The model under review builds one solid part; all positions refer to its coordinate system, in mm. A direction names the side the tool comes from. Round coordinates to 2 decimals unless told otherwise and drop trailing zeros. Write each loop counter-clockwise with the first axis right and the second up, starting at its lowest first coordinate (ties: lowest second). Pieces come first, ordered by that corner, then holes. Notation, with made-up numbers: M -22,21 L 26,21 A30 ccw 26,44 Z; hole C 7,12.25 d3. An arc over 180 degrees is marked long. One line per item, written item: value. Start each with the question number.
1) Take a section at B-B, the plane x = 3. Write out the cut boundary in (y, z), and give its area (3 significant figures).
2) Take a section at D-D, the plane z = 11. Write out the cut boundary in (x, y).
3) Tool access review of faces 1 (the face through (0, 60, -1)), 2 (the face through (1.054, 15.789, -13.672)), 3 (the face through (-4.6, 45.07, 17.19)), 4 (the face through (0, 43, -15)), 5 (the face through (2, 30, 16)): name each direction out of +Z, -Z, +X, -X, +Y, -Y from which nothing blocks a thin tool from reaching the whole face with its end or side.
4) Mouldability with a two-part tool opening along X and no side actions: class faces 6 (the face through (0, 15, -21)), 7 (the face through (10, 31, -1)), 8 (the face through (0.05, 23.03, -6.25)) as +X half, -X half, draft (parallel to the pull), parting line (faces both ways), or undercut.
5) Wall thickness on probe 1 along X at (y, z) = (59, -5); probe 2 along Y at (x, z) = (8.75, 10); probe 3 along X at (y, z) = (57, -6): over which ranges is each line inside the solid? List them lowest first.
6) Take a section at C-C, the plane z = -8. Write out the cut boundary in (x, y), and give its area (3 significant figures).
7) For P1, Ø6.5, axis at x = 0, z = -5, coming from the +Y side; P2, Ø2, axis at x = 4, y = 47.5, coming from the -Z side; P3, Ø1.5, axis at x = 0, z = -13, coming from the -Y side; P4, Ø5, axis at x = 3, y = 45, coming from the -Z side, all flat-tipped, find the tip position at first contact; note any pin that passes through.
8) Take a section at A-A, the plane y = 10. Write out the cut boundary in (x, z).
from build123d import *

# Parameters (mm, degrees)
BOSS_EXTRUDE1_DEPTH     = 10
SKETCH2_R               = 7
CUT_EXTRUDE1_DEPTH      = 67.219332525
M3_TAPPED_HOLE1_D       = 2.5
M3_TAPPED_HOLE1_DEPTH   = 8.248924226
M3_TAPPED_HOLE1_TIP     = 0.751075774
CUT_EXTRUDE2_DEPTH      = 2
SKETCH7_R               = 2
CUT_EXTRUDE3_DEPTH      = 30
SKETCH8_R               = 1.25
CUT_EXTRUDE4_DEPTH      = 49
CUT_EXTRUDE5_REACH      = 76.458
CUT_EXTRUDE5_END_RADIUS = 7
SKETCH9_R               = 1.6
SKETCH10_R              = 2.5
CUT_EXTRUDE6_DEPTH      = 69.447059925
CUT_EXTRUDE7_REACH      = 68.219
CUT_EXTRUDE7_END_RADIUS = 2.5
SKETCH11_R              = 1.25
CUT_EXTRUDE8_REACH      = 68.219
SKETCH12_R              = 4
M4_TAPPED_HOLE1_D       = 3.3
M4_TAPPED_HOLE1_DEPTH   = 9.008579979
M4_TAPPED_HOLE1_TIP     = 0.991420021


with BuildPart() as part:
    # Sketch1 → Boss-Extrude1 (new, symmetric)
    with BuildSketch(Plane(origin=(0, 0, 0), x_dir=(0, 0, -1), z_dir=(1, 0, 0))):
        Polygon((0, 0), (0, 30), (-19, 30), (-19, 62), (9, 62), (21, 24), (21, 0), align=None)
    extrude(amount=BOSS_EXTRUDE1_DEPTH, both=True)

    # Sketch2 → Cut-Extrude1 (cut, through all)
    with BuildSketch(Plane(origin=(0, 62, 0), x_dir=(1, 0, 0), z_dir=(0, 1, 0))):
        with Locations(Location((0, -9, 0), (0, 0, 270))):
            Circle(SKETCH2_R)
    extrude(amount=-CUT_EXTRUDE1_DEPTH, mode=Mode.SUBTRACT)

    # M3 Tapped Hole1
    with Locations(Plane(origin=(0, 62, 0), x_dir=(1, 0, 0), z_dir=(0, 1, 0))):
        with Locations((-7, -16), (7, -16), (7, 5), (-7, 5)):
            Hole(M3_TAPPED_HOLE1_D / 2, depth=M3_TAPPED_HOLE1_DEPTH)
            with Locations((0, 0, -(M3_TAPPED_HOLE1_DEPTH + M3_TAPPED_HOLE1_TIP / 2))):  # 118° drill point
                Cone(0, M3_TAPPED_HOLE1_D / 2, M3_TAPPED_HOLE1_TIP, mode=Mode.SUBTRACT)

    # Sketch6 → Cut-Extrude2 (cut)
    with BuildSketch(Plane(origin=(0, 62, 0), x_dir=(1, 0, 0), z_dir=(0, 1, 0))):
        with BuildLine():
            Line((2, 5), (2, -4.41407825))
            ThreePointArc((2, -4.41407825), (0, -6.41407825), (-2, -4.41407825))
            Line((-2, -4.41407825), (-2, 5))
            ThreePointArc((-2, 5), (0, 7), (2, 5))
        make_face()
    extrude(amount=-CUT_EXTRUDE2_DEPTH, mode=Mode.SUBTRACT)

    # Sketch7 → Cut-Extrude3 (cut)
    with BuildSketch(Plane(origin=(0, 62, 0), x_dir=(1, 0, 0), z_dir=(0, 1, 0))):
        with Locations(Location((0, 5, 0), (0, 0, 270))):
            Circle(SKETCH7_R)
    extrude(amount=-CUT_EXTRUDE3_DEPTH, mode=Mode.SUBTRACT)

    # Sketch8 → Cut-Extrude4 (cut)
    with BuildSketch(Plane(origin=(0, 62, 0), x_dir=(1, 0, 0), z_dir=(0, 1, 0))):
        with Locations(Location((0, 5, 0), (0, 0, 270))):
            Circle(SKETCH8_R)
    extrude(amount=-CUT_EXTRUDE4_DEPTH, mode=Mode.SUBTRACT)

    # Cut-Extrude5: up to this cylinder (the profile starts outside it)
    cut_extrude5_end = Plane(origin=(0, 45, 9), z_dir=(0, 1, 0)) * Cylinder(CUT_EXTRUDE5_END_RADIUS, 167.916, mode=Mode.PRIVATE)
    # Sketch9 → Cut-Extrude5 (cut, up to the surface)
    with BuildSketch(Plane.XY.offset(19), mode=Mode.PRIVATE) as cut_extrude5_sk1:
        with Locations((-3, 45)):
            Circle(SKETCH9_R)
    cut_extrude5_tool1 = extrude(cut_extrude5_sk1.sketch, amount=-CUT_EXTRUDE5_REACH, mode=Mode.PRIVATE) - cut_extrude5_end
    add(cut_extrude5_tool1.solids().sort_by_distance((-3, 45, 19))[0], mode=Mode.SUBTRACT)
    # Sketch9 → Cut-Extrude5 (cut, up to the surface)
    with BuildSketch(Plane.XY.offset(19), mode=Mode.PRIVATE) as cut_extrude5_sk2:
        with Locations((3, 45)):
            Circle(SKETCH9_R)
    cut_extrude5_tool2 = extrude(cut_extrude5_sk2.sketch, amount=-CUT_EXTRUDE5_REACH, mode=Mode.PRIVATE) - cut_extrude5_end
    add(cut_extrude5_tool2.solids().sort_by_distance((3, 45, 19))[0], mode=Mode.SUBTRACT)

    # Sketch10 → Cut-Extrude6 (cut, through all)
    with BuildSketch(Plane(origin=(10, 0, 0), x_dir=(0, 0, -1), z_dir=(1, 0, 0))):
        with Locations((13, 20)):
            Circle(SKETCH10_R)
    extrude(amount=-CUT_EXTRUDE6_DEPTH, mode=Mode.SUBTRACT)

    # Cut-Extrude7: up to this cylinder (the profile starts outside it)
    cut_extrude7_end = Plane(origin=(0, 20, -13), z_dir=(1, 0, 0)) * Cylinder(CUT_EXTRUDE7_END_RADIUS, 142.438, mode=Mode.PRIVATE)
    # Sketch11 → Cut-Extrude7 (cut, up to the surface)
    with BuildSketch(Plane.XZ, mode=Mode.PRIVATE) as cut_extrude7_sk1:
        with Locations(Location((0, -13, 0), (0, 0, 270))):
            Circle(SKETCH11_R)
    cut_extrude7_tool1 = extrude(cut_extrude7_sk1.sketch, amount=-CUT_EXTRUDE7_REACH, mode=Mode.PRIVATE) - cut_extrude7_end
    add(cut_extrude7_tool1.solids().sort_by_distance((0, 0, -13))[0], mode=Mode.SUBTRACT)

    # Sketch12 → Cut-Extrude8 (cut, up to next)
    with BuildSketch(Plane.XY, mode=Mode.PRIVATE) as cut_extrude8_sk1:
        with Locations((0, 10)):
            Circle(SKETCH12_R)
    cut_extrude8_tool1 = extrude(cut_extrude8_sk1.sketch, amount=-CUT_EXTRUDE8_REACH, mode=Mode.PRIVATE) & part.part
    add(cut_extrude8_tool1.solids().sort_by_distance((0, 10, 0))[0], mode=Mode.SUBTRACT)

    # M4 Tapped Hole1
    with Locations(Plane(origin=(0, 0, 0), x_dir=(-1, 0, 0), z_dir=(0, -1, 0))):
        with Locations((0, 13), (0, 5)):
            Hole(M4_TAPPED_HOLE1_D / 2, depth=M4_TAPPED_HOLE1_DEPTH)
            with Locations((0, 0, -(M4_TAPPED_HOLE1_DEPTH + M4_TAPPED_HOLE1_TIP / 2))):  # 118° drill point
                Cone(0, M4_TAPPED_HOLE1_D / 2, M4_TAPPED_HOLE1_TIP, mode=Mode.SUBTRACT)


solid = part.part
Checked values:
1. outline: M 0,-21 L 7.35,-21 L 7.35,0 L 0,0 Z; M 12.65,-21 L 24,-21 L 62,-9 L 62,2.68 L 30,2.68 L 30,0 L 12.65,0 Z; M 30,15.32 L 43.4,15.32 L 43.4,19 L 30,19 Z; M 46.6,15.32 L 62,15.32 L 62,19 L 46.6,19 Z; hole C 20,-13 d5
1. area: 1,130 mm2
2. outline: M -10,30 L -6.71,30 L -6.71,62 L -10,62 Z; M 6.71,30 L 10,30 L 10,62 L 6.71,62 Z
3. face 1: +Y
3. face 2: -Y
3. face 3: +Z
3. face 4: -Z, +X, -X, +Y
3. face 5: +Z, +X, -X, -Y
4. face 6: draft
4. face 7: +X half
4. face 8: undercut
5. probe 1: x = -10 to -8.25, -5.75 to -2, 2 to 5.75, 8.25 to 10
5. probe 2: y = 30 to 62
5. probe 3: x = -10 to -7.75, -6.25 to -1.73, 1.73 to 6.25, 7.75 to 10
6. outline: M -10,0 L 10,0 L 10,62 L -10,62 Z; hole C 0,10 d8
6. area: 1,190 mm2
7. P1: stops at y = 62
7. P2: stops at z = -13.89
7. P3: stops at y = 22.38
7. P4: stops at z = -15.16
8. outline: M -10,-21 L -4,-21 L -4,0 L -10,0 Z; M 4,-21 L 10,-21 L 10,0 L 4,0 Z
